Could you check a few things on this model? Use its own coordinates, in mm. Face numbers are marked on the shaded views. A direction names the side the tool comes from. Coordinates: 2 decimals unless noted, no trailing zeros. Order: outer loops, then holes, each group sorted by start corner. A loop starts at its lowest first (then second) coordinate and runs counter-clockwise, first axis right, second up. Notation, with made-up numbers: M 6,53.25 L 41,53.25 A10 cw 41,69.25 Z; hole C 55,31 d2. An arc over 180 degrees is marked long. One line per question, with ' | ' between items. Start each with the question number.
from build123d import *

# Parameters (mm, degrees)
F0_W     = 30
F0_H     = 91
F1_DEPTH = 2
F2_W     = 30
F2_H     = 91
F2_W_2   = 24
F2_H_2   = 86
F3_DEPTH = 32
F4_R     = 2
F5_DEPTH = 25
F7_DEPTH = 20


with BuildPart() as f1:
    # F0 (on Top) → F1 (new body)
    with BuildSketch(Plane.XY):
        with Locations((2.462509, 0.307451)):
            Rectangle(F0_W, F0_H)
    extrude(amount=F1_DEPTH)

    # F2 (on face) → F3 (join)
    with BuildSketch(Plane.XY.offset(2)):
        with Locations((2.462509, 0.307451)):
            Rectangle(F2_W, F2_H)
        with Locations((2.462509, -0.192549)):
            Rectangle(F2_W_2, F2_H_2, mode=Mode.SUBTRACT)
    extrude(amount=F3_DEPTH)

    # F4 (on face) → F5 (cut)
    with BuildSketch(Plane(origin=(-12.537491, 0, 0), x_dir=(0, -1, 0), z_dir=(-1, 0, 0))):
        with Locations((-20.091893, 30)):
            Circle(F4_R)
        with Locations((19.908107, 30)):
            Circle(F4_R)
    extrude(amount=-F5_DEPTH, mode=Mode.SUBTRACT)

    # F6 (on face) → F7 (cut)
    with BuildSketch(Plane.XY.offset(34)):
        Polygon((-12.537491, 45.807451), (-12.537491, 25.807451), (-9.537491, 25.807451), (-9.537491, 42.807451), (14.462509, 42.807451), (14.462509, -43.192549), (-9.537491, -43.192549), (-9.537491, -25.192549), (-12.537491, -25.192549), (-12.537491, -45.192549), (17.462509, -45.192549), (17.462509, 45.807451), align=None)
    extrude(amount=-F7_DEPTH, mode=Mode.SUBTRACT)


solid = f1.part
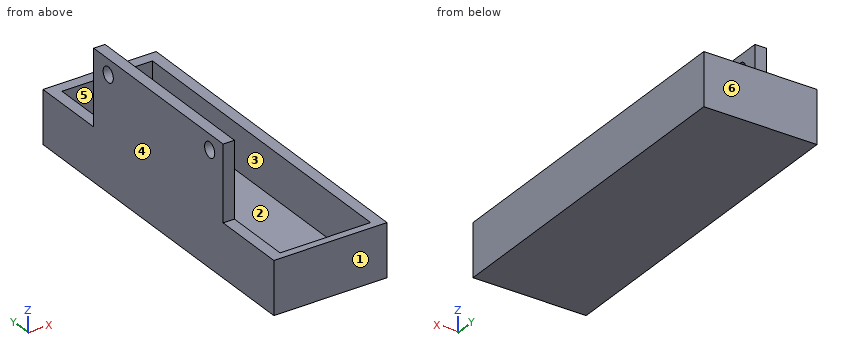
(1) Imagine slicing it at C-C, the plane x = 9.5. Write out the boundary of the cut face in (y, z), plus the area to 3 significant figures.
(2) Imagine slicing it at B-B, the plane y = 39.5. Write out the boundary of the cut face in (x, z).
(3) We'd pull the mould along X, two halves only. Please class the marked faces 1, 2, 3 and 4: +X half, -X half, draft (parallel to the pull), parting line (faces both ways), or undercut.
(4) Imagine slicing it at A-A, the plane z = 30. Write out the boundary of the cut face in (x, y).
(5) For P1, Ø2, axis at x = -2.5, y = -32, coming from the +Z side; P2, Ø1, axis at x = -4.5, y = 3.5, coming from the -Z side; P3, Ø3.5, axis at x = -10.5, z = 19.5, coming from the -Y side; P4, Ø3.5, axis at x = -11, z = 27.5, coming from the +Y side, each with a flat end and sliding along its axis, tell me the tip position at first contact or that it passes through.
(6) Imagine slicing it at D-D, the plane z = 15. Write out the boundary of the cut face in (x, y), plus the area to 3 significant figures.
(7) On a 3-axis mill with a long thin cutter (end or side, diameter ignored), from which of +Z, -Z, +X, -X, +Y, -Y can I reach the whole of each face in a straight line? I mean the marked faces 5 and 6. Say none if no direction works.
(8) If I drill on line 1 along Z through (x, y) = (5, -27); line 2 along Y through (x, z) = (7.25, 9); line 3 along X through (y, z) = (-39.5, 12.5), over which ranges is the centre line in solid material (lowest first)? Write a range as from..to.
Answers:
1) outline: M -45.19,0 L 45.81,0 L 45.81,14 L 42.81,14 L 42.81,2 L -43.19,2 L -43.19,14 L -45.19,14 Z | area: 242 mm²
2) outline: M -12.54,0 L 17.46,0 L 17.46,14 L 14.46,14 L 14.46,2 L -9.54,2 L -9.54,14 L -12.54,14 Z
3) face 1: draft | face 2: undercut | face 3: undercut | face 4: -X half
4) outline: M -12.54,-25.19 L -9.54,-25.19 L -9.54,-21.91 L -12.54,-21.91 Z; M -12.54,-17.91 L -9.54,-17.91 L -9.54,18.09 L -12.54,18.09 Z; M -12.54,22.09 L -9.54,22.09 L -9.54,25.81 L -12.54,25.81 Z
5) P1: z = 2 | P2: z = 0 | P3: y = -25.19 | P4: y = 25.81
6) outline: M -12.54,-25.19 L -9.54,-25.19 L -9.54,25.81 L -12.54,25.81 Z | area: 153 mm²
7) face 5: +Z | face 6: +Z, -Z, +X, -X, +Y
8) line 1: 0..2 | line 2: -45.19..-43.19, 42.81..45.81 | line 3: -12.54..-9.54, 14.46..17.46
